Check sheet for the modelled part. Datum: model origin and axes. Units: mm. A direction names the side the tool comes from. Round coordinates to 2 decimals unless told otherwise and drop trailing zeros. Write each loop counter-clockwise with the first axis right and the second up, starting at its lowest first coordinate (ties: lowest second). Pieces come first, ordered by that corner, then holes. Notation, with made-up numbers: (-38.75, 76.25) - (-6.75, 76.25) arc R15 cw to (-6.75, 90.25) - close; hole circle Ø1 at (31.25, 74). An arc over 180 degrees is marked (long way). Answer as a JSON object with one key per item and string values. Group by question number.
Item 1: Thickness scan on line 1 (Y direction, x = 44, z = 7.75); line 2 (X direction, y = -29, z = 16); line 3 (Z direction, x = 29, y = -26) (3 decimals). Record the ranges inside material, lowest first.
Item 2: Sectioned sample at C-C on z = 9.25. Record the boundary of the cut face in (x, y) (3 decimals).
Item 3: Sectioned sample at A-A on x = -44.45. Record the boundary of the cut face in (y, z) (3 decimals).
Item 4: Set-up check for faces 1 (the cylindrical face through (-27.733, -9.518, 9.891)), 2 (the flat face through (29, -24, 13.335)), 3 (the cylindrical face through (17.83, -12.89, 9.39)), 4 (the flat face through (15.2, 0.3, 9.4)), 5 (the cylindrical face through (-68.23, -21.7, 9.39)): record each of +Z, -Z, +X, -X, +Y, -Y from which the full face is reachable in a straight line by a thin tool's end or side.
Item 5: Sectioned sample at B-B on y = 7. Record the boundary of the cut face in (x, z), plus the area to 3 significant figures.
Item 6: Release check for a two-part mould opening along X. For faces 6 (the flat face through (-1, -9, 0)), 7 (the flat face through (-49, -22, 6.35)) record: pulls with the +X half, pulls with the -X half, needs draft (parallel to the pull), parting line crosses it, or undercut.
Item 7: Gauge pin test, flat ends, axial feed: P1, Ø2, axis at y = -27.5, z = 15, coming from the +X side; P2, Ø1.5, axis at x = 32.5, z = 7, coming from the -Y side; P3, Ø1, axis at x = 54, z = 16, coming from the -Y side (3 decimals). Record the tip position at first contact, or that the pin passes through.
```python
from build123d import *

# Parameters (mm, degrees)
PAD_DEPTH       = 19.05
SKETCH001_R     = 17.526
POCKET_DEPTH    = 12.7
SKETCH002_R     = 6.985
POCKET001_DEPTH = 6.351
CHAMFER_SIZE    = 1.27
SKETCH003_R     = 20.32
POCKET002_DEPTH = 3.175


with BuildPart() as part:
    # Sketch → Pad (new body)
    with BuildSketch(Plane.XY):
        with BuildLine():
            ThreePointArc((-26.517355, 2.297173), (-67.949508, -22.598065), (-19.859908, -17.720926))
            ThreePointArc((-13.408051, -9.812702), (-17.782581, -12.829737), (-19.859908, -17.720926))
            Line((-10.685782, -8.907353), (-13.408051, -9.812702))
            ThreePointArc((-3.932394, -9.188814), (-7.283282, -8.428887), (-10.685782, -8.907353))
            ThreePointArc((-3.932394, -9.188814), (0, -9.9949), (3.932394, -9.188814))
            ThreePointArc((10.685782, -8.907353), (7.283282, -8.428887), (3.932394, -9.188814))
            Line((10.685782, -8.907353), (13.408051, -9.812702))
            ThreePointArc((19.859908, -17.720926), (17.782581, -12.829737), (13.408051, -9.812702))
            ThreePointArc((19.859908, -17.720926), (67.949508, -22.598065), (26.517355, 2.297173))
            ThreePointArc((16.614313, -0.171878), (21.924443, -0.375685), (26.517355, 2.297173))
            Line((13.892044, 0.73347), (16.614313, -0.171878))
            ThreePointArc((8.652348, 5.003488), (10.880692, 2.388068), (13.892044, 0.73347))
            ThreePointArc((8.652348, 5.003488), (0, 9.9949), (-8.652348, 5.003488))
            ThreePointArc((-13.892044, 0.73347), (-10.880692, 2.388068), (-8.652348, 5.003488))
            Line((-13.892044, 0.73347), (-16.614313, -0.171878))
            ThreePointArc((-26.517355, 2.297173), (-21.924443, -0.375685), (-16.614313, -0.171878))
        make_face()
    extrude(amount=PAD_DEPTH)

    # Sketch001 (on Face18 of Pad) → Pocket (cut)
    with BuildSketch(Plane.XY.offset(19.05)):
        with Locations((-44.45, -14.7828)):
            Circle(SKETCH001_R)
        with Locations((44.45, -14.7828)):
            Circle(SKETCH001_R)
    extrude(amount=-POCKET_DEPTH, mode=Mode.SUBTRACT)

    # Sketch002 (on Face21 of Pocket) → Pocket001 (cut, through all)
    with BuildSketch(Plane.XY.offset(6.35)):
        with Locations((-44.45, -14.7828)):
            Circle(SKETCH002_R)
        with Locations((44.45, -14.7828)):
            Circle(SKETCH002_R)
    extrude(amount=-POCKET001_DEPTH, mode=Mode.SUBTRACT)

    # Chamfer
    chamfer_edges = [part.edges().sort_by_distance(p)[0] for p in [
        (-51.435, -14.7828, 6.35),
        (37.465, -14.7828, 6.35),
    ]]
    chamfer(chamfer_edges, length=CHAMFER_SIZE)

    # Sketch003 (on DatumPlane) → Pocket002 (cut)
    with BuildSketch(Plane.XY.offset(13.335)):
        with Locations((-44.45, -14.7828)):
            Circle(SKETCH003_R)
        with Locations((44.45, -14.7828)):
            Circle(SKETCH003_R)
    extrude(amount=POCKET002_DEPTH, mode=Mode.SUBTRACT)


solid = part.part
```
Completed:
{
 "1": {"line 1": "-39.54 to -32.3, 2.74 to 9.98", "line 2": "-64.73 to -58.97, -29.93 to -24.17, 24.17 to 29.93, 58.97 to 64.73", "line 3": "0 to 13.335, 16.51 to 19.05"},
 "2": {"outline": "(-26.517, 2.297) arc R24.765 ccw (long way) to (-19.86, -17.721) arc R9.525 cw to (-13.408, -9.813) - (-10.686, -8.907) arc R9.525 cw to (-3.932, -9.189) arc R9.995 ccw to (3.932, -9.189) arc R9.525 cw to (10.686, -8.907) - (13.408, -9.813) arc R9.525 cw to (19.86, -17.721) arc R24.765 ccw (long way) to (26.517, 2.297) arc R9.525 cw to (16.614, -0.172) - (13.892, 0.733) arc R9.525 cw to (8.652, 5.003) arc R9.995 ccw to (-8.652, 5.003) arc R9.525 cw to (-13.892, 0.733) - (-16.614, -0.172) arc R9.525 cw to start; hole circle Ø35.052 at (-44.45, -14.783); hole circle Ø35.052 at (44.45, -14.783)"},
 "3": {"outline": "(-39.548, 0) - (-21.768, 0) - (-21.768, 5.08) - (-23.038, 6.35) - (-32.309, 6.35) - (-32.309, 13.335) - (-35.103, 13.335) - (-35.103, 16.51) - (-32.309, 16.51) - (-32.309, 19.05) - (-39.548, 19.05) - close; (-7.798, 0) - (9.982, 0) - (9.982, 19.05) - (2.743, 19.05) - (2.743, 16.51) - (5.537, 16.51) - (5.537, 13.335) - (2.743, 13.335) - (2.743, 6.35) - (-6.528, 6.35) - (-7.798, 5.08) - close"},
 "4": {"face 1": "+Z", "face 2": "none", "face 3": "+Z, -Z, -Y", "face 4": "+Z, -Z, +Y", "face 5": "+Z, -Z"},
 "5": {"outline": "(-56.23, 0) - (-32.67, 0) - (-32.67, 19.05) - (-56.23, 19.05) - close; (-7.13, 0) - (7.13, 0) - (7.13, 19.05) - (-7.13, 19.05) - close; (32.67, 0) - (56.23, 0) - (56.23, 19.05) - (32.67, 19.05) - close", "area": "1,170 mm²"},
 "6": {"face 6": "needs draft", "face 7": "undercut"},
 "7": {"P1": "x = 66.27", "P2": "y = -36.87", "P3": "y = -37.835"}
}
